Geometry: see drawing. Coordinates: mm, zero at the bounding-box minimum. Coordinates: 2 decimals unless noted, no trailing zeros. Loops run counter-clockwise (first coordinate to the right, second up) from the corner with the lowest first, then second, coordinate; pieces in that order, holes last. Notation, with made-up numbers: (-31.75, -30) - (-10.75, -30) arc R17 cw to (-10.75, -2) - close; hole circle Ø6 at (47, 32). An arc over 180 degrees is marked (long way). Write each question's results on one line, items separated by ' | '. Start each with the question number.
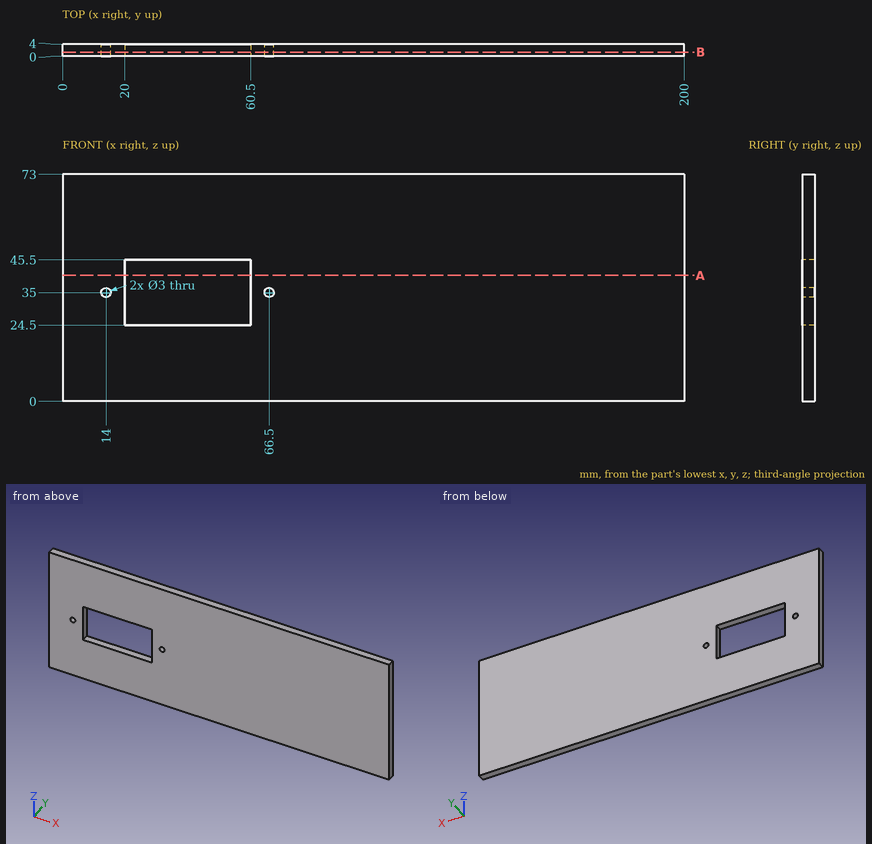
1) Material intervals for line 1 (X direction, y = 2.3, z = 35); line 2 (Z direction, x = 14, y = 2.8); line 3 (X direction, y = 1.2, z = 26.5), sorted ascending. Write a range as [from, to].
2) Section query A-A on z = 40.5. Output: boundary loops of the cut face in (x, y), and give its area (3 significant figures).
3) Pin query (flat end, axial travel): pin 1 Ø2.5 at (x, z) = (14, 35) entering from +Y. Return the tip coordinate at first contact, or that it passes through.
4) Section query B-B on y = 1.35. Output: boundary loops of the cut face in (x, z), and give its area (3 significant figures).
Returned:
1) line 1: x = [0, 12.5], [15.5, 20], [60.5, 65], [68, 200] | line 2: z = [0, 33.5], [36.5, 73] | line 3: x = [0, 20], [60.5, 200]
2) outline: (0, 0) - (20, 0) - (20, 4) - (0, 4) - close; (60.5, 0) - (200, 0) - (200, 4) - (60.5, 4) - close | area: 638 mm²
3) pin 1: passes through
4) outline: (0, 0) - (200, 0) - (200, 73) - (0, 73) - close; hole circle Ø3 at (14, 35); hole (20, 24.5) - (60.5, 24.5) - (60.5, 45.5) - (20, 45.5) - close; hole circle Ø3 at (66.5, 35) | area: 13,700 mm²
